Design review of the part built by this model. Coordinates are the model's own, in mm. A direction names the side the tool comes from. Coordinates: 2 decimals unless noted, no trailing zeros. Write each loop counter-clockwise with the first axis right and the second up, starting at its lowest first coordinate (ties: lowest second). Pieces come first, ordered by that corner, then holes. Notation, with made-up numbers: (-34.75, 74.25) - (-1.75, 74.25) arc R17 ccw to (-1.75, 89.25) - close; hole circle Ø8 at (20.5, 28.5). An arc over 180 degrees is marked (long way). Answer as a JSON object with one key per item and string values.
```python
from build123d import *

# Parameters (mm, degrees)
SKETCH2_W           = 45
SKETCH2_H           = 80
BOSS_EXTRUDE2_DEPTH = 35
SHELL2_T            = 3
SKETCH5_R           = 4
CUT_EXTRUDE1_DEPTH  = 3
SKETCH6_R           = 4
CUT_EXTRUDE2_DEPTH  = 3
SKETCH7_W           = 12
SKETCH7_H           = 40
CUT_EXTRUDE3_DEPTH  = 3
SKETCH8_W           = 50
SKETCH8_H           = 12
CUT_EXTRUDE4_DEPTH  = 3
FILLET1_R           = 3
FILLET2_R           = 3


with BuildPart() as part:
    # Sketch2 → Boss-Extrude2 (new body)
    with BuildSketch(Plane(origin=(0, 0, 0), x_dir=(1, 0, 0), z_dir=(0, 1, 0))):
        with Locations((22.5, -40)):
            Rectangle(SKETCH2_W, SKETCH2_H)
    extrude(amount=BOSS_EXTRUDE2_DEPTH)

    # Shell2
    shell2_openings = [part.faces().sort_by_distance(p)[0] for p in [
        (22.5, 17.5, 0),
        (22.5, 17.5, 80),
    ]]
    offset(amount=SHELL2_T, openings=shell2_openings, kind=Kind.INTERSECTION)

    # Sketch5 → Cut-Extrude1 (cut)
    with BuildSketch(Plane(origin=(0, 38, 0), x_dir=(1, 0, 0), z_dir=(0, 1, 0))):
        with Locations(Location((20, -70, 0), (0, 0, 270))):
            Circle(SKETCH5_R)
        with Locations(Location((20, -10, 0), (0, 0, 270))):
            Circle(SKETCH5_R)
        Polygon((32, 0), (32, -20), (7, -20), (7, -60), (32, -60), (32, -80), (48, -80), (48, 0), align=None)
    extrude(amount=-CUT_EXTRUDE1_DEPTH, mode=Mode.SUBTRACT)

    # Sketch6 → Cut-Extrude2 (cut)
    with BuildSketch(Plane(origin=(48, 0, 0), x_dir=(0, 0, -1), z_dir=(1, 0, 0))):
        with Locations((-70, 7)):
            Circle(SKETCH6_R)
        with Locations((-10, 7)):
            Circle(SKETCH6_R)
        Polygon((-80, 15), (-60, 15), (-60, -3), (-20, -3), (-20, 15), (0, 15), (0, 35), (-80, 35), align=None)
    extrude(amount=-CUT_EXTRUDE2_DEPTH, mode=Mode.SUBTRACT)

    # Sketch7 → Cut-Extrude3 (cut)
    with BuildSketch(Plane.XZ.offset(3)):
        with Locations((42, 40)):
            Rectangle(SKETCH7_W, SKETCH7_H)
    extrude(amount=-CUT_EXTRUDE3_DEPTH, mode=Mode.SUBTRACT)

    # Sketch8 → Cut-Extrude4 (cut)
    with BuildSketch(Plane.ZY.offset(3)):
        with Locations((40, 13)):
            Rectangle(SKETCH8_W, SKETCH8_H)
    extrude(amount=-CUT_EXTRUDE4_DEPTH, mode=Mode.SUBTRACT)

    # Fillet1
    fillet1_edges = [part.edges().sort_by_distance(p)[0] for p in [
        (36, -1.5, 60),
        (36, -1.5, 20),
        (0, 0, 40),
        (45, 0, 70),
        (0, 35, 40),
        (7, 36.5, 60),
        (7, 36.5, 20),
        (-3, 38, 40),
        (48, -3, 70),
        (-3, -3, 40),
        (45, 0, 10),
        (48, -3, 10),
    ]]
    fillet(fillet1_edges, radius=FILLET1_R - 0.0001)  # a hair under: the kernel refuses the full size

    # Fillet2
    fillet2_edges = [part.edges().sort_by_distance(p)[0] for p in [
        (-1.5, 7, 65),
        (-1.5, 19, 65),
        (-1.5, 19, 15),
        (-1.5, 7, 15),
    ]]
    fillet(fillet2_edges, radius=FILLET2_R)


solid = part.part
```
(1) Take a section at C-C, the plane x = 27. Write out the cut boundary in (y, z).
Solved:
{"outline": "(-3, 0) - (0, 0) - (0, 80) - (-3, 80) - close; (35, 0) - (38, 0) - (38, 20) - (35, 20) - close; (35, 60) - (38, 60) - (38, 80) - (35, 80) - close"}
(2) Tool access review of faces 5 (the face through (21, 37, 60)), 6 (the face through (47, 15, 10)), 7 (the face through (4, 35, 39)): name each direction out of +Z, -Z, +X, -X, +Y, -Y from which nothing blocks a thin tool from reaching the whole face with its end or side.
Solved:
{"face 5": "+X, +Y", "face 6": "+Z, -Z, +X, +Y", "face 7": "+Z, -Z, +X"}
(3) Take a section at D-D, the plane x = 20. Write out the cut boundary in (y, z), and give its area (3 significant figures).
Solved:
{"outline": "(-3, 0) - (0, 0) - (0, 80) - (-3, 80) - close; (35, 0) - (38, 0) - (38, 6) - (35, 6) - close; (35, 14) - (38, 14) - (38, 20) - (35, 20) - close; (35, 60) - (38, 60) - (38, 66) - (35, 66) - close; (35, 74) - (38, 74) - (38, 80) - (35, 80) - close", "area": "312 mm^2"}
(4) Take a section at B-B, the plane z = 10. Give the number of separate pieces and of enclosed holes in the cut face, and give its area (3 significant figures).
Solved:
{"separate pieces": "3", "enclosed holes": "0", "area": "360 mm^2"}
(5) To check wall thickness, follow line 1 (X direction, y = 27, z = 71.5); line 2 (X direction, y = 36, z = 70); line 3 (X direction, y = 3, z = 12). State the ranges of each line that lie inside material, in increasing order. Write a range as from..to.
Solved:
{"line 1": "x = -3..0", "line 2": "x = -2.83..16, 24..32", "line 3": "x = -3..0, 45..48"}
(6) The part is to be moulded in two halves that separate along Y. For faces 1 (the face through (7.9, 36.48, 20.86)), 2 (the face through (44.1, 0.86, 69.86)), 3 (the face through (-1.48, 18.14, 15.9)), 4 (the face through (47, 7, 14)), say which applies: pulls with the +Y half, pulls with the -Y half, needs draft (parallel to the pull), parting line crosses it, or undercut.
Solved:
{"face 1": "needs draft", "face 2": "pulls with the +Y half", "face 3": "undercut", "face 4": "undercut"}
(7) Take a section at A-A, the plane y = 12.5. Write out the cut boundary in (x, z), and give its area (3 significant figures).
Solved:
{"outline": "(-3, 0) - (0, 0) - (0, 15) - (-3, 15) - close; (-3, 65) - (0, 65) - (0, 80) - (-3, 80) - close; (45, 0) - (48, 0) - (48, 20) - (45, 20) - close; (45, 60) - (48, 60) - (48, 80) - (45, 80) - close", "area": "210 mm^2"}
(8) For pin 1 (10 mm diameter, centred on x = 40.5, z = 36, fed in from +Y); pin 2 (19.5 mm diameter, centred on x = 23, z = 22.5, fed in from +Y); pin 3 (0.9 mm diameter, centred on x = 46, z = 9.5, fed in from +Y); pin 4 (1.5 mm diameter, centred on x = -1, z = 41.5, fed in from -Y), all flat-tipped, find the tip position at first contact; note any pin that passes through.
Solved:
{"pin 1": "stops at y = 0", "pin 2": "stops at y = 38", "pin 3": "stops at y = 15", "pin 4": "stops at y = -2.99"}
